Geometry check sheet. Reference: drawing and pictorial views, mm from the part's lowest x, y, z. A direction names the side the tool comes from. Coordinates: 2 decimals unless noted, no trailing zeros. Write each loop counter-clockwise with the first axis right and the second up, starting at its lowest first coordinate (ties: lowest second). Pieces come first, ordered by that corner, then holes. Notation, with made-up numbers: (13, 69) -> (63, 69) arc R21 cw to (63, 80) -> close; hole circle Ø7 at (82.25, -12). An arc over 180 degrees is marked (long way). Use a Markdown table: item, result.
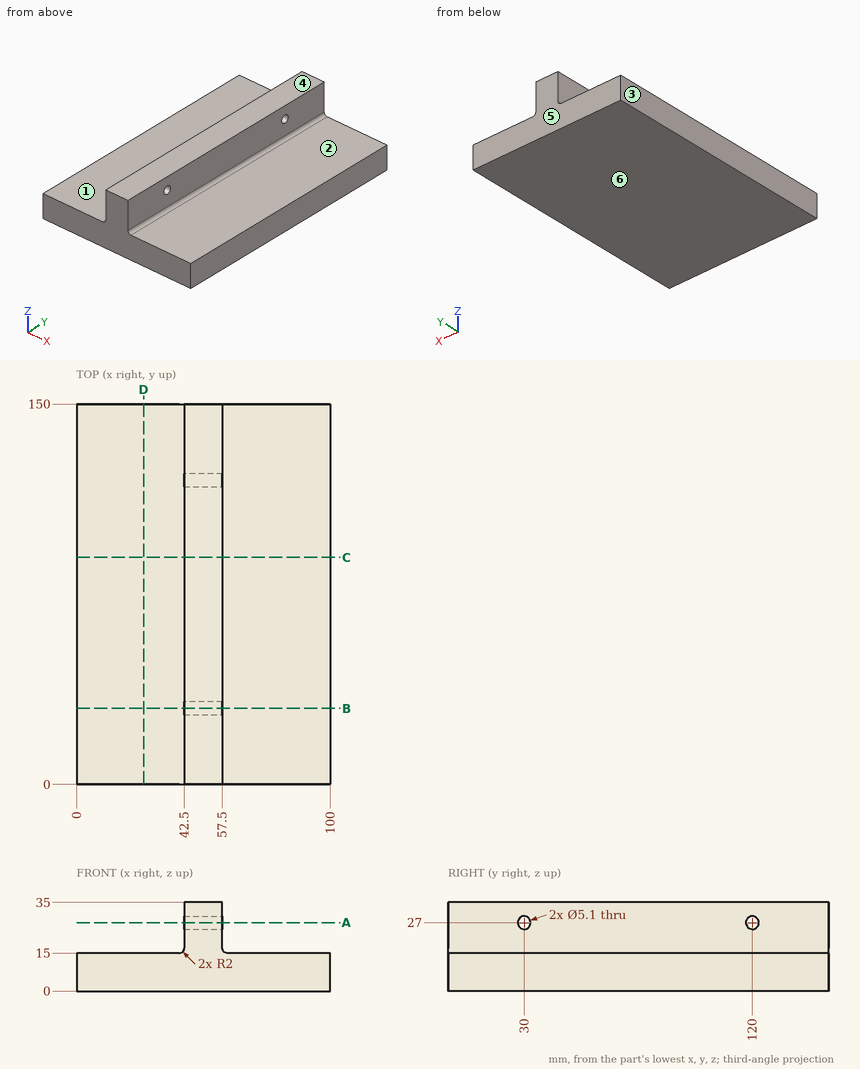
Item 1: Section check C-C on y = 89.5. Record the boundary of the cut face in (x, z).
Answer block:
| item | result |
|---|---|
| outline | (0, 0) -> (100, 0) -> (100, 15) -> (59.5, 15) arc R2 cw to (57.5, 17) -> (57.5, 35) -> (42.5, 35) -> (42.5, 17) arc R2 cw to (40.5, 15) -> (0, 15) -> close |
Item 2: Tool access check on the marked faces 1, 2 and 3. Record the directions out of +Z, -Z, +X, -X, +Y, -Y that give a thin tool (end or side, any length) a straight path to the whole face; none if there is none.
Answer block:
| item | result |
|---|---|
| face 1 | +Z, -X, +Y, -Y |
| face 2 | +Z, +X, +Y, -Y |
| face 3 | +Z, -Z, -X, +Y, -Y |
Item 3: Mould release check, pull along Z, two halves, no side actions. Record for the marked faces 4, 5 and 6: +Z half, -Z half, draft (parallel to the pull), parting line (faces both ways), or undercut.
Answer block:
| item | result |
|---|---|
| face 4 | +Z half |
| face 5 | draft |
| face 6 | -Z half |
Item 4: Section check B-B on y = 30. Record the boundary of the cut face in (x, z), then the cut area to 3 significant figures.
Answer block:
| item | result |
|---|---|
| outline | (0, 0) -> (100, 0) -> (100, 15) -> (59.5, 15) arc R2 cw to (57.5, 17) -> (57.5, 24.45) -> (42.5, 24.45) -> (42.5, 17) arc R2 cw to (40.5, 15) -> (0, 15) -> close; (42.5, 29.55) -> (57.5, 29.55) -> (57.5, 35) -> (42.5, 35) -> close |
| area | 1,730 mm^2 |
Item 5: Thickness scan on L1, parallel to Z at x = 51.25, y = 30; L2, parallel to Z at x = 18.5, y = 46.5; L3, parallel to X at y = 130, z = 33.5. Record the ranges inside material, lowest first. Write a range as [from, to].
Answer block:
| item | result |
|---|---|
| L1 | z = [0, 24.45], [29.55, 35] |
| L2 | z = [0, 15] |
| L3 | x = [42.5, 57.5] |
Item 6: Section check A-A on z = 27. Record the boundary of the cut face in (x, y).
Answer block:
| item | result |
|---|---|
| outline | (42.5, 0) -> (57.5, 0) -> (57.5, 27.45) -> (42.5, 27.45) -> close; (42.5, 32.55) -> (57.5, 32.55) -> (57.5, 117.45) -> (42.5, 117.45) -> close; (42.5, 122.55) -> (57.5, 122.55) -> (57.5, 150) -> (42.5, 150) -> close |
Item 7: Section check D-D on x = 26.5. Record the boundary of the cut face in (y, z), then the cut area to 3 significant figures.
Answer block:
| item | result |
|---|---|
| outline | (0, 0) -> (150, 0) -> (150, 15) -> (0, 15) -> close |
| area | 2,250 mm^2 |
Item 8: Depth check by flat-ended pin: P1, Ø14.5, axis at y = 42.5, z = 25, coming from the -X side; P2, Ø5, axis at y = 35, z = 27.5, coming from the +X side. Enter the tip coordinate at first touch or a pass-through.
Answer block:
| item | result |
|---|---|
| P1 | stops at x = 42.5 |
| P2 | stops at x = 57.5 |
